Can you work these out from the model? Positions are in its coordinate system, mm. Coordinates: 2 decimals unless noted, no trailing zeros. Order: outer loops, then holes, each group sorted by start corner. A loop starts at its lowest first (then second) coordinate and runs counter-clockwise, first axis right, second up. Notation, with made-up numbers: (24.25, 81.25) -> (55.25, 81.25) arc R28 ccw to (55.25, 110.25) -> close; hole circle Ø4 at (62.25, 5). An arc over 180 degrees is marked (long way). Answer as a JSON object with one key per item and string values. Group by question number.
(1) I need wall thicknesses on line 1 (Y direction, x = 20.5, z = 19). Which ranges of the line are inside material? Lowest first, please.
(2) I want a section at B-B, the plane x = -15.5. List the corners of the cut face in (y, z) for me.
(3) If we mould it in two halves opening along X, with no side actions, what happens to faces 1 (the flat face through (-2, 18, 15)), 2 (the cylindrical face through (-33.211, 9.126, 30.905)), 3 (the flat face through (29.649, 9, 15)), 4 (the flat face through (-24, 19, 15))? For each: pulls with the +X half, pulls with the -X half, needs draft (parallel to the pull), parting line crosses it, or undercut.
(4) I want a section at C-C, the plane z = 0. List the corners of the cut face in (x, y) for me, plus the area to 3 significant figures.
(5) For pin 1 (0.5 mm diameter, centred on x = 5.5, y = 18.5, fed in from +Z); pin 2 (0.8 mm diameter, centred on y = 18.5, z = 13, fed in from +X); pin 3 (0.8 mm diameter, centred on x = -8.5, y = 18.5, fed in from -Z), each with a flat end and sliding along its axis, tell me the tip position at first contact or that it passes through.
(6) I want a section at A-A, the plane z = 21. List the corners of the cut face in (x, y) for me, plus the area to 3 significant figures.
Autodesk Inventor part; units mm, degrees
ref_plane "YZ Plane" through (0, 0, 0) normal (1, 0, 0) x (0, 1, 0)
ref_plane "XZ Plane" through (0, 0, 0) normal (0, 1, 0) x (-1, 0, 0)
ref_plane "XY Plane" through (0, 0, 0) normal (0, 0, 1) x (1, 0, 0)
sketch "Sketch1" plane through (0, 0, 0) normal (0, 1, 0) x (-1, 0, 0)
  line L0 (34.3512, 32.1074) -> (-29.6488, 32.1074)
  line L1 (-29.6488, 32.1074) -> (-29.6488, -2.8926)
  line L2 (-29.6488, -2.8926) -> (34.3512, -2.8926)
  line L3 (34.3512, -2.8926) -> (34.3512, 32.1074)
  line L4 (27.3512, 26.6074) -> (20.3512, 26.6074)
  line L5 (20.3512, 26.6074) -> (20.3512, 2.6074)
  line L6 (20.3512, 2.6074) -> (27.3512, 2.6074)
  line L7 (27.3512, 2.6074) -> (27.3512, 26.6074)
  line L8 (13.3512, 2.6074) -> (13.3512, 26.6074)
  line L9 (13.3512, 26.6074) -> (6.3512, 26.6074)
  line L10 (6.3512, 2.6074) -> (13.3512, 2.6074)
  line L11 (6.3512, 26.6074) -> (6.3512, 2.6074)
  line L12 (-0.6488, 2.6074) -> (-0.6488, 26.6074)
  line L13 (-0.6488, 26.6074) -> (-7.6488, 26.6074)
  line L14 (-7.6488, 2.6074) -> (-0.6488, 2.6074)
  line L15 (-7.6488, 26.6074) -> (-7.6488, 2.6074)
  point P0 (0, 0)
  dimension "d0" = 35
  dimension "d1" = 64
  dimension "d2" = 7
  dimension "d3" = 7
  dimension "d4" = 24
  dimension "d5" = 5.5
  dimension "d6" = 5.5
  dimension "d9" = 14
  dimension "d14" = 7
extrude "Extrusion1" add sketch "Sketch1" along normal blind 18
extrude "Extrusion2" add sketch "Sketch1" along normal blind 19 contours L7 L6 L5 L4 | L10 L11 L9 L8 | L14 L15 L13 L12
fillet "Fillet1" radius 4 4 edges at (-34.3512, 9, -2.8926) (-34.3512, 9, 32.1074) (29.6488, 9, -2.8926) (29.6488, 9, 32.1074)
properties part number "kluc"
Computed values:
{
 "1": {"line 1": "y = 0 to 18"},
 "2": {"outline": "(0, -2.89) -> (18, -2.89) -> (18, 32.11) -> (0, 32.11) -> close"},
 "3": {"face 1": "undercut", "face 2": "pulls with the -X half", "face 3": "pulls with the +X half", "face 4": "needs draft"},
 "4": {"outline": "(-34.19, 0) -> (29.49, 0) -> (29.49, 18) -> (-34.19, 18) -> close", "area": "1,150 mm2"},
 "5": {"pin 1": "stops at z = 26.61", "pin 2": "stops at x = 7.65", "pin 3": "stops at z = 2.61"},
 "6": {"outline": "(-34.35, 0) -> (29.65, 0) -> (29.65, 18) -> (7.65, 18) -> (7.65, 19) -> (0.65, 19) -> (0.65, 18) -> (-6.35, 18) -> (-6.35, 19) -> (-13.35, 19) -> (-13.35, 18) -> (-20.35, 18) -> (-20.35, 19) -> (-27.35, 19) -> (-27.35, 18) -> (-34.35, 18) -> close", "area": "1,170 mm2"}
}
